Autodesk Inventor part; units mm, degrees
ref_plane "YZ Plane" through (0, 0, 0) normal (1, 0, 0) x (0, 1, 0)
ref_plane "XZ Plane" through (0, 0, 0) normal (0, 1, 0) x (-1, 0, 0)
ref_plane "XY Plane" through (0, 0, 0) normal (0, 0, 1) x (1, 0, 0)
sketch "Sketch1" plane through (0, 0, 0) normal (0, 1, 0) x (-1, 0, 0)
  circle A0 centre (0, 0) radius 150
  circle A1 centre (-13.3087, -279.6835) radius 100
  circle A2 centre (-424.1378, -546.7404) radius 100
  line L0 (0, 0) -> (-13.3087, -279.6835)
  line L1 (-13.3087, -279.6835) -> (-424.1378, -546.7404)
  line L2 (-424.1378, -546.7404) -> (-1339.0994, -538.3521)
  arc A3 (-1324.0769, -381.4083) -> (-1301.514, -806.4251) centre (-424.1378, -546.7404) ccw
  line L3 (25.7594, -1.2258) -> (11.8229, -294.1053)
  line L4 (11.8229, -294.1053) -> (-416.6006, -572.5992)
  line L5 (-416.6006, -572.5992) -> (-1338.9723, -564.1429)
  arc A4 (25.7594, -1.2258) -> (0, 0) centre (12.8797, -0.6129) ccw
  dimension "d0" = 300
  dimension "d1" = 200
  dimension "d2" = 200
  dimension "d3" = 490
  dimension "d4" = 280
  dimension "d10" = 915
extrude "Extrusion1" add sketch "Sketch1" along normal blind 100
properties part number "95thMaleTemplate"
Read the model definition and answer for the solid it produces. Units are mm, in the model's axes. Round coordinates to 2 decimals unless told otherwise and drop trailing zeros. Write each loop counter-clockwise with the first axis right and the second up, starting at its lowest first coordinate (ties: lowest second). Pieces come first, ordered by that corner, then holes. Notation, with made-up numbers: M -12.5,64 L 1.5,64 A14 cw 1.5,82 Z; hole C 56,21.5 d4. An arc over 180 degrees is marked long. One line per item, written item: value.
Q1. Find section A-A on y = 24. Write down the section's boundary in (x, z), plus the area to 3 significant figures.
Data:
outline: M -18.74,-148.83 L -17.04,-184.4 A100 ccw long 80.26,-353.96 L 329.08,-515.7 A100 ccw long 520.99,-571.64 L 1338.97,-564.14 A915 ccw 1339.1,-538.35 L 524.13,-545.82 A100 ccw 340.3,-492.24 L 97.15,-334.18 A100 ccw 8.56,-179.8 L 7.13,-149.83 A150 ccw long Z
area: 163,000 mm2
Q2. Find section C-C on x = 1136. Write down the section's boundary in (y, z), plus the area to 3 significant figures.
Data:
outline: M 0,-566 L 100,-566 L 100,-540.21 L 0,-540.21 Z
area: 2,580 mm2
Q3. For a pull along X with two mould halves and no side action, classify faces 1 (the flat face through (217.021, 49.3, -412.106)), 2 (the flat face through (7.833, 49.3, -164.604)), 3 (the flat face through (-17.9, 49.3, -166.4)), 4 (the cylindrical face through (-74.641, 49.3, -327.275)) as +X half, -X half, draft (parallel to the pull), parting line (faces both ways), or undercut.
Data:
face 1: undercut
face 2: +X half
face 3: -X half
face 4: undercut
Q4. Straight lines are drawn through the part: line 1 (Z direction, x = -59, y = 49); line 2 (Z direction, x = 57, y = 73.5); line 3 (Z direction, x = 1236.5, y = 33.5). For each, find the intervals that lie inside material, in ascending order. Write a range as [from, to].
Data:
line 1: [-348.76, -210.61], [-137.91, 137.91]
line 2: [-369.63, -189.73], [-138.75, 138.75]
line 3: [-565.08, -539.29]
Q5. Flat-ended cylindrical pins translate along their axes: pin 1 Ø1.5 at (x, y) = (877.5, 81.5) entering from -Z; pin 2 Ø3 at (x, y) = (674, 78) entering from -Z; pin 3 Ø8 at (y, z) = (20, -355) entering from -X. Find the tip coordinate at first contact, or state that the pin passes through.
Data:
pin 1: z = -568.38
pin 2: z = -570.25
pin 3: x = -56.79
Q6. Find section B-B on z = 0. Write down the section's boundary in (x, y).
Data:
outline: M -150,0 L 150,0 L 150,100 L -150,100 Z
